from build123d import *

# Parameters (mm, degrees)
CROQUIS1_W              = 20
CROQUIS1_H              = 14
SALIENTE_EXTRUIR1_DEPTH = 32.8
CROQUIS2_W              = 20
CROQUIS2_H              = 27.8
CORTAR_EXTRUIR2_DEPTH   = 10
REDONDEO1_R             = 4
CROQUIS3_R              = 1.9
CORTAR_EXTRUIR3_DEPTH   = 36


with BuildPart() as part:
    # Croquis1 → Saliente-Extruir1 (new body)
    with BuildSketch(Plane.XY):
        Rectangle(CROQUIS1_W, CROQUIS1_H)
    extrude(amount=SALIENTE_EXTRUIR1_DEPTH)

    # Croquis2 → Cortar-Extruir2 (cut)
    with BuildSketch(Plane(origin=(0, 7, 0), x_dir=(1, 0, 0), z_dir=(0, 1, 0))):
        with Locations((0, -16.4)):
            Rectangle(CROQUIS2_W, CROQUIS2_H)
    extrude(amount=-CORTAR_EXTRUIR2_DEPTH, mode=Mode.SUBTRACT)

    # Redondeo1
    redondeo1_edges = [part.edges().sort_by_distance(p)[0] for p in [
        (0, -3, 2.5),
        (0, -3, 30.3),
    ]]
    fillet(redondeo1_edges, radius=REDONDEO1_R)

    # Croquis3 → Cortar-Extruir3 (cut)
    with BuildSketch(Plane(origin=(0, 0, 0), x_dir=(-1, 0, 0), z_dir=(0, 0, -1))):
        with Locations((0, -1)):
            Circle(CROQUIS3_R)
    extrude(amount=-CORTAR_EXTRUIR3_DEPTH, mode=Mode.SUBTRACT)


solid = part.part
Source: CAD feature listing. Evaluate the final solid. Frame: model axes, mm. A direction names the side the tool comes from. Give positions to 0.01 mm unless a question says otherwise; leave off trailing zeros. Write each loop counter-clockwise with the first axis right and the second up, starting at its lowest first coordinate (ties: lowest second). Pieces come first, ordered by that corner, then holes. Notation, with made-up numbers: M -18.75,71 L 35.25,71 A26 ccw 35.25,93 Z; hole C -19,87 d10. An arc over 180 degrees is marked long. Return JSON: item names as keys, results as strings. Group by question number.
1) Ray query, L1, parallel to Z at x = 5.5, y = 2.75; L2, parallel to Y at x = 0, z = 31.3; L3, parallel to X at y = -1, z = 29.85. Return the intervals inside material, ascending.
2) Cut plane A-A, the plane y = -1.5. Output: boundary loops of the cut face in (x, z), then the cut area to 3 significant figures.
3) Cut plane D-D, the plane x = -5. Output: boundary loops of the cut face in (y, z).
4) Set-up query: faces 4 (the face through (0, 2, 0)), 5 (the face through (-2.082, -1.859, 29.097)). Return all of +Z, -Z, +X, -X, +Y, -Y with unobstructed straight access to the full face (end or side cutting, diameter ignored); none if empty.
5) First-contact query: pin 1 Ø1.5 at (x, z) = (8, 13.5) entering from +Y; pin 2 Ø3.5 at (x, y) = (0, -1) entering from -Z. Flat tips, straight axial feed; report the tip coordinate or a pass-through.
6) Cut plane B-B, the plane y = 1.75. Output: boundary loops of the cut face in (x, z).
7) Draft query along Y for faces 1 (the face through (0, 4, 2.5)), 2 (the face through (0, 7, 1)), 3 (the face through (0.412, -2.855, 30.579)). Return one class per face: released by +Y, released by -Y, zero draft, split by the parting line, or undercut.
8) Cut plane C-C, the plane x = 0. Output: boundary loops of the cut face in (y, z), then the cut area to 3 significant figures.
Data:
{
 "1": {"L1": "z = 0 to 2.5, 30.3 to 32.8", "L2": "y = -7 to -2.9, 0.9 to 7", "L3": "x = -10 to -1.9, 1.9 to 10"},
 "2": {"outline": "M -10,0 L -1.83,0 L -1.83,3.38 L -10,3.38 Z; M -10,29.42 L -1.83,29.42 L -1.83,32.8 L -10,32.8 Z; M 1.83,0 L 10,0 L 10,3.38 L 1.83,3.38 Z; M 1.83,29.42 L 10,29.42 L 10,32.8 L 1.83,32.8 Z", "area": "110 mm²"},
 "3": {"outline": "M -7,0 L 7,0 L 7,2.5 L 1,2.5 A4 cw -3,6.5 L -3,26.3 A4 cw 1,30.3 L 7,30.3 L 7,32.8 L -7,32.8 Z"},
 "4": {"face 4": "-Z, +X, -X, +Y, -Y", "face 5": "+X, -X, +Y"},
 "5": {"pin 1": "stops at y = -3", "pin 2": "passes through"},
 "6": {"outline": "M -10,0 L 10,0 L 10,2.5 L -10,2.5 Z; M -10,30.3 L 10,30.3 L 10,32.8 L -10,32.8 Z"},
 "7": {"face 1": "zero draft", "face 2": "released by +Y", "face 3": "undercut"},
 "8": {"outline": "M -7,0 L -2.9,0 L -2.9,5.61 A4 cw -3,6.5 L -3,26.3 A4 cw -2.9,27.19 L -2.9,32.8 L -7,32.8 Z; M 0.9,0 L 7,0 L 7,2.5 L 1,2.5 A4 cw 0.9,2.5 Z; M 0.9,30.3 A4 cw 1,30.3 L 7,30.3 L 7,32.8 L 0.9,32.8 Z", "area": "163 mm²"}
}
